Verification items for the finished model (mm, model axes). Round coordinates to 2 decimals unless told otherwise and drop trailing zeros. Order: outer loops, then holes, each group sorted by start corner. A loop starts at its lowest first (then second) coordinate and runs counter-clockwise, first axis right, second up. Notation, with made-up numbers: (33, 5) -> (89, 5) arc R12 ccw to (89, 13) -> close; hole circle Ø6 at (-6, 59). An arc over 180 degrees is marked (long way). Put each result on its own line as item: value.
Autodesk Inventor part; units mm, degrees
ref_plane "YZ Plane" through (0, 0, 0) normal (1, 0, 0) x (0, 1, 0)
ref_plane "XZ Plane" through (0, 0, 0) normal (0, 1, 0) x (-1, 0, 0)
ref_plane "XY Plane" through (0, 0, 0) normal (0, 0, 1) x (1, 0, 0)
sketch "Sketch1" plane through (0, 0, 0) normal (0, 1, 0) x (-1, 0, 0)
  line L0 (408.912, 674) -> (-408.912, 674)
  line L1 (-458.912, 624) -> (-458.912, -624)
  line L2 (-408.912, -674) -> (408.912, -674)
  line L3 (458.912, -624) -> (458.912, 624)
  line L4 (458.912, 674) -> (-458.912, -674) construction
  line L5 (408.912, 674) -> (408.912, 624)
  line L6 (408.912, 624) -> (458.912, 624)
  line L7 (458.912, 674) -> (408.912, 624) construction
  line L8 (408.912, 674) -> (458.912, 624) construction
  line L9 (-458.912, 624) -> (-408.912, 624)
  line L10 (-408.912, 624) -> (-408.912, 674)
  line L11 (-408.912, 674) -> (-458.912, 624) construction
  line L12 (-458.912, 674) -> (-408.912, 624) construction
  line L13 (458.912, -624) -> (408.912, -624)
  line L14 (408.912, -624) -> (408.912, -674)
  line L15 (458.912, -624) -> (408.912, -674) construction
  line L16 (408.912, -624) -> (458.912, -674) construction
  line L17 (-408.912, -624) -> (-458.912, -624)
  line L18 (-408.912, -674) -> (-408.912, -624)
  line L19 (-408.912, -624) -> (-458.912, -674) construction
  line L20 (-458.912, -624) -> (-408.912, -674) construction
  point P0 (0, 0)
  point P1 (433.912, 649)
  point P2 (-433.912, 649)
  point P3 (433.912, -649)
  point P4 (-433.912, -649)
extrude "Extrusion1" add sketch "Sketch1" along normal blind 20
sketch "Sketch2" plane through (0, 20, 0) normal (0, 1, 0) x (1, 0, 0)
  line L0 (452, 602) -> (-452, 602)
  line L1 (-452, -602) -> (452, -602)
  line L2 (452, 602) -> (-452, -602) construction
  line L3 (-452, 602) -> (452, -602) construction
  line L4 (452, 622) -> (-452, 622)
  line L5 (-452, -622) -> (452, -622)
  line L6 (452, 622) -> (-452, -622) construction
  line L7 (-452, 622) -> (452, -622) construction
  line L8 (452, -622) -> (452, -602)
  line L9 (452, 602) -> (452, 622)
  line L10 (-452, 622) -> (-452, 602)
  line L11 (-452, -602) -> (-452, -622)
  point P0 (0, 0)
extrude "Extrusion2" add sketch "Sketch2" along normal blind 20
properties part number "tub floor 2"
Item 1: Gauge pin test, flat ends, axial feed: pin 1 Ø22 at (y, z) = (10, -642) entering from +X; pin 2 Ø2 at (x, y) = (-71.5, 22) entering from +Z; pin 3 Ø22 at (y, z) = (33.5, 612.5) entering from +X. Record the tip position at first contact, or that the pin passes through.
Check sheet entries:
pin 1: stops at x = 408.91
pin 2: stops at z = 622
pin 3: stops at x = 452
Item 2: Material ranges on L1, parallel to Z at x = -6, y = 25; L2, parallel to Y at x = -156, z = 169, recorded low to high. Write a range as [from, to].
Check sheet entries:
L1: z = [-622, -602], [602, 622]
L2: y = [0, 20]
Item 3: Release check for a two-part mould opening along Z. For faces 1 (the flat face through (6, 0, 9)), 2 (the flat face through (6, 20, -140)) record: +Z half, -Z half, draft (parallel to the pull), parting line (faces both ways), or undercut.
Check sheet entries:
face 1: draft
face 2: undercut
Item 4: Section check C-C on z = -462. Record the boundary of the cut face in (x, y).
Check sheet entries:
outline: (-458.91, 0) -> (458.91, 0) -> (458.91, 20) -> (-458.91, 20) -> close
Item 5: Section check B-B on x = 229. Record the boundary of the cut face in (y, z).
Check sheet entries:
outline: (0, -674) -> (20, -674) -> (20, -622) -> (40, -622) -> (40, -602) -> (20, -602) -> (20, 602) -> (40, 602) -> (40, 622) -> (20, 622) -> (20, 674) -> (0, 674) -> close
Item 6: Section check A-A on y = 29. Record the boundary of the cut face in (x, z), then the cut area to 3 significant figures.
Check sheet entries:
outline: (-452, -622) -> (452, -622) -> (452, -602) -> (-452, -602) -> close; (-452, 602) -> (452, 602) -> (452, 622) -> (-452, 622) -> close
area: 36,200 mm^2
